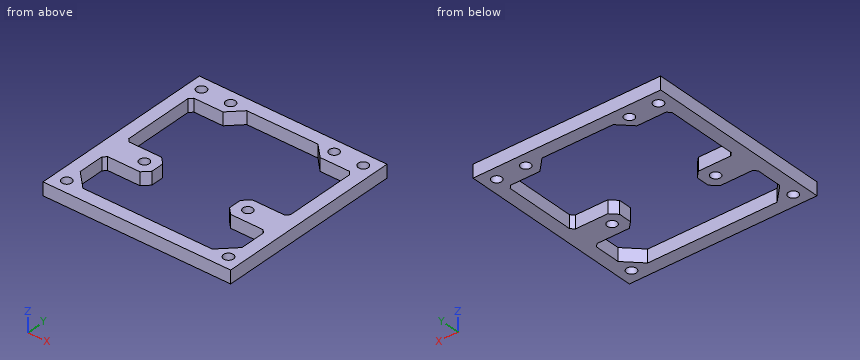
```python
from build123d import *

# Parameters (mm, degrees)
SKETCH009_W     = 58
SKETCH009_H     = 58
SKETCH009_R     = 1.525
SKETCH009_R_2   = 1.5
PAD005_DEPTH    = 4
CHAMFER_SIZE    = 2
CHAMFER001_SIZE = 1


with BuildPart() as part:
    # Sketch009 → Pad005 (new body)
    with BuildSketch(Plane.XY):
        Rectangle(SKETCH009_W, SKETCH009_H)
        with Locations((-25, 25)):
            Circle(SKETCH009_R, mode=Mode.SUBTRACT)
        with Locations((25, 25)):
            Circle(SKETCH009_R, mode=Mode.SUBTRACT)
        with Locations((25, -25)):
            Circle(SKETCH009_R, mode=Mode.SUBTRACT)
        with Locations((-25, -25)):
            Circle(SKETCH009_R, mode=Mode.SUBTRACT)
        with Locations((-16, 25)):
            Circle(SKETCH009_R_2, mode=Mode.SUBTRACT)
        with Locations((16, 25)):
            Circle(SKETCH009_R_2, mode=Mode.SUBTRACT)
        with Locations((-16, -7)):
            Circle(SKETCH009_R_2, mode=Mode.SUBTRACT)
        with Locations((16, -7)):
            Circle(SKETCH009_R_2, mode=Mode.SUBTRACT)
        Polygon((-25, -3), (-12, -3), (-12, -11), (-25, -11), (-25, -20), (-20, -25), (20, -25), (25, -20), (25, -11), (12, -11), (12, -3), (25, -3), (25, 21), (15, 21), (11, 25), (-11, 25), (-15, 21), (-25, 21), align=None, mode=Mode.SUBTRACT)
    extrude(amount=PAD005_DEPTH)

    # Chamfer
    chamfer_edges = [part.edges().sort_by_distance(p)[0] for p in [
        (-12, -3, 2),
        (-12, -11, 2),
        (12, -11, 2),
        (12, -3, 2),
    ]]
    chamfer(chamfer_edges, length=CHAMFER_SIZE)

    # Chamfer001
    chamfer001_edges = [part.edges().sort_by_distance(p)[0] for p in [
        (-25, -3, 2),
        (-25, 21, 2),
        (25, 21, 2),
        (25, -3, 2),
        (-25, -11, 2),
        (25, -11, 2),
    ]]
    chamfer(chamfer001_edges, length=CHAMFER001_SIZE)


solid = part.part
```
Part model, mm, in its own coordinate system. Coordinates: 2 decimals unless noted, no trailing zeros. Loops run counter-clockwise (first coordinate to the right, second up) from the corner with the lowest first, then second, coordinate; pieces in that order, holes last. Notation, with made-up numbers: (-31.5, 78) - (-15.5, 78) arc R15 cw to (-15.5, 103) - close; hole circle Ø6 at (60, 75). An arc over 180 degrees is marked (long way). Write item = value, one per line. Start each with the question number.
Item 1: Cut at A-A, the plane x = 16. Give the cut face in (y, z), and give its area (3 significant figures).
Item 2: Cut at B-B, the plane y = 1. Give the cut face in (x, z), and give its area (3 significant figures).
Item 3: Wall check: L1, parallel to Y at x = 16, z = 1.85; L2, parallel to Y at x = 10, z = 1.9. Give the ranges that are in metal, low to high. Write a range as from..to.
Item 4: Cut at C-C, the plane y = -7. Give the cut face in (x, z), and give its area (3 significant figures).
The answers:
q1.outline = (-29, 0) - (-25, 0) - (-25, 4) - (-29, 4) - close; (-11, 0) - (-8.5, 0) - (-8.5, 4) - (-11, 4) - close; (-5.5, 0) - (-3, 0) - (-3, 4) - (-5.5, 4) - close; (21, 0) - (23.5, 0) - (23.5, 4) - (21, 4) - close; (26.5, 0) - (29, 0) - (29, 4) - (26.5, 4) - close
q1.area = 56.0 mm2
q2.outline = (-29, 0) - (-25, 0) - (-25, 4) - (-29, 4) - close; (25, 0) - (29, 0) - (29, 4) - (25, 4) - close
q2.area = 32.0 mm2
q3.L1 = -29..-25, -11..-8.5, -5.5..-3, 21..23.5, 26.5..29
q3.L2 = -29..-25, 25..29
q4.outline = (-29, 0) - (-17.5, 0) - (-17.5, 4) - (-29, 4) - close; (-14.5, 0) - (-12, 0) - (-12, 4) - (-14.5, 4) - close; (12, 0) - (14.5, 0) - (14.5, 4) - (12, 4) - close; (17.5, 0) - (29, 0) - (29, 4) - (17.5, 4) - close
q4.area = 112 mm2
